Job drawing, mm, ordinate dimensions from the low corner. One solid piece. A direction names the side the tool comes from. Round coordinates to 2 decimals unless told otherwise and drop trailing zeros. Loops run counter-clockwise (first coordinate to the right, second up) from the corner with the lowest first, then second, coordinate; pieces in that order, holes last. Notation, with made-up numbers: M 2.25,-4.5 L 53.25,-4.5 A17 cw 53.25,11.5 Z; hole C 31.25,75 d4. An arc over 180 degrees is marked long. Use one line per item in the form item = value.
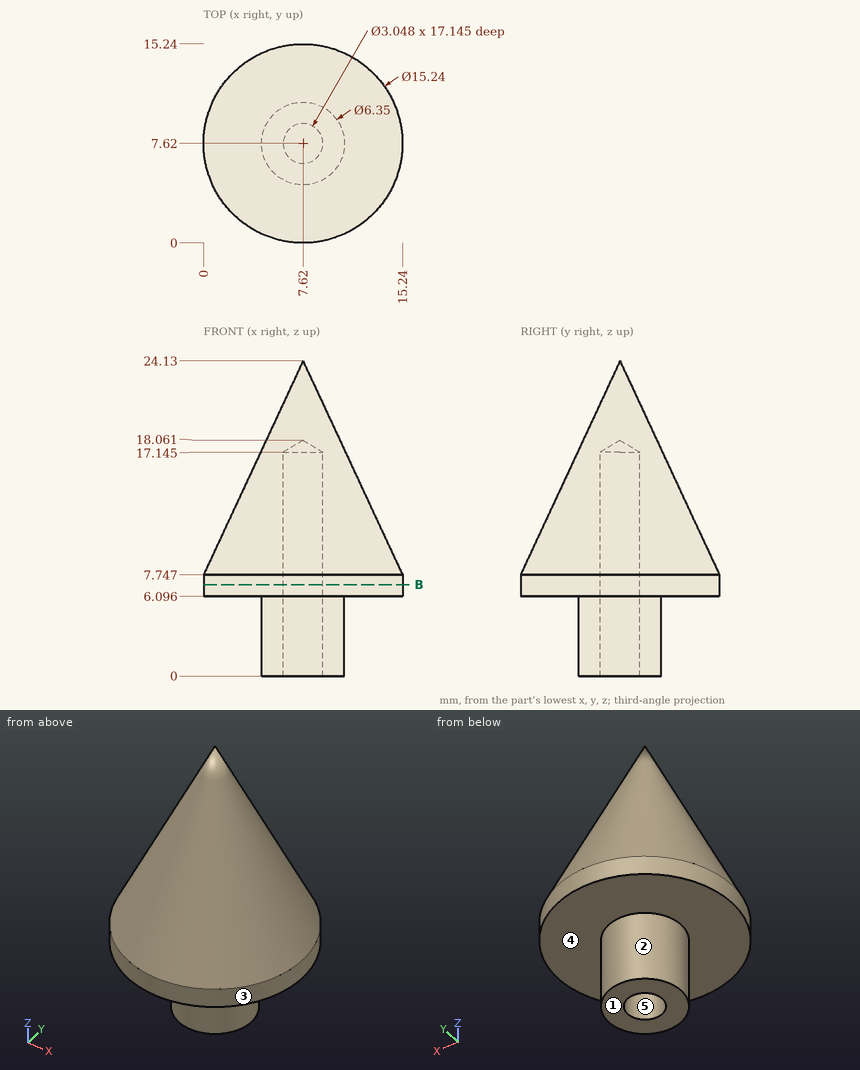
1. Cut at B-B on z = 7. Write the cut outline in (x, y).
Completed:
outline = C 7.62,7.62 d15.24; hole C 7.62,7.62 d3.05
2. Probe line 1 along Y through (x, z) = (7.62, 4.25) (1 decimal); line 2 along X through (y, z) = (8.5, 13.5) (1 decimal); line 3 along Z through (x, y) = (13, 11) (1 decimal). List the from-to ranges inside material, lowest first. Write a range as from..to.
Completed:
line_1 = 4.4..6.1, 9.1..10.8
line_2 = 2.8..6.4, 8.9..12.5
line_3 = 6.1..10.5
3. Drop flat-ended pins along their axis: P1, Ø1.5, axis at x = 12, y = 4.5, coming from the +Z side; P2, Ø2, axis at x = 2, y = 2.5, coming from the +Z side (1 decimal); P3, Ø1, axis at y = 4.5, z = 9.5, coming from the -X side. Give the stop position or say it passes through.
Completed:
P1 = 14.18
P2 = 9.9
P3 = 1.22
4. Tool access for the marked faces 1 and 2: list every direction of +Z, -Z, +X, -X, +Y, -Y with a clear straight run to the whole face (end or side of a thin tool).
Completed:
face_1 = -Z, +X, -X, +Y, -Y
face_2 = -Z
5. Pull direction X, two halves, no side cores. Call the marked faces 3, 4 and 5: +X half, -X half, draft (parallel to the pull), parting line (faces both ways), or undercut.
Completed:
face_3 = parting line
face_4 = draft
face_5 = undercut
